Source: CAD feature listing. Evaluate the final solid. Frame: model axes, mm. A direction names the side the tool comes from. Give positions to 0.01 mm unless a question says otherwise; leave off trailing zeros. Loops run counter-clockwise (first coordinate to the right, second up) from the corner with the lowest first, then second, coordinate; pieces in that order, holes last. Notation, with made-up numbers: (43, 41) -> (89, 41) arc R12 ccw to (89, 57) -> close; hole circle Ø3 at (57.5, 22). An arc over 180 degrees is marked (long way). Return JSON: item names as keys, results as strings. Group by question number.
```python
from build123d import *

# Parameters (mm, degrees)
F4_T     = -1.2
F5_SIZE  = 0.5
F6_W     = 3.6
F6_H     = 11.6
F7_DEPTH = 5


with BuildPart() as f3:
    # F2 (on offset) → F3 section 0
    with BuildSketch(Plane.XY.offset(165)):
        with BuildLine():
            Line((-64, -36), (64, -36))
            ThreePointArc((64, -36), (89.4558441227, -25.4558441227), (100, 0))
            ThreePointArc((100, 0), (89.4558441227, 25.4558441227), (64, 36))
            Line((64, 36), (-64, 36))
            ThreePointArc((-64, 36), (-89.4558441227, 25.4558441227), (-100, 0))
            ThreePointArc((-100, 0), (-89.4558441227, -25.4558441227), (-64, -36))
        make_face()
    # F0 (on Top) → F3 section 1
    with BuildSketch(Plane.XY):
        with BuildLine():
            Line((-64, -36), (64, -36))
            ThreePointArc((64, -36), (89.4558441227, -25.4558441227), (100, 0))
            ThreePointArc((100, 0), (89.4558441227, 25.4558441227), (64, 36))
            Line((64, 36), (-64, 36))
            ThreePointArc((-64, 36), (-89.4558441227, 25.4558441227), (-100, 0))
            ThreePointArc((-100, 0), (-89.4558441227, -25.4558441227), (-64, -36))
        make_face()
    loft()

    # F4
    f4_openings = [f3.faces().sort_by_distance(p)[0] for p in [
        (0, 0, 0),
    ]]
    offset(amount=F4_T, openings=f4_openings)

    # F5
    f5_edges = [f3.edges().sort_by_distance(p)[0] for p in [
        (-100, 0, 165),
        (0, 36, 165),
        (100, 0, 165),
        (0, -36, 165),
        (-98.8, 0, 163.8),
        (0, -34.8, 163.8),
        (98.8, 0, 163.8),
        (0, 34.8, 163.8),
    ]]
    chamfer(f5_edges, length=F5_SIZE)

    # F6 (on face) → F7 (join)
    with BuildSketch(Plane(origin=(0, 0, 163.8), x_dir=(1, 0, 0), z_dir=(0, 0, -1))):
        Rectangle(F6_W, F6_H)
    extrude(amount=F7_DEPTH)


solid = f3.part
```
1) Mould query, pull axis X, two halves, no side actions, for faces 3 (the face through (1, 36, 81)), 4 (the face through (-1, -34.8, 81)), 5 (the face through (1, 8, 163.8)). Classes: released by +X, released by -X, zero draft, split by the parting line, or undercut.
2) Contact query for flat-ended pins moving along their axis: P1, Ø2, axis at x = 71, y = -8, coming from the -Z side; P2, Ø1, axis at y = 26.5, z = 102, coming from the +X side; P3, Ø1, axis at y = -10.5, z = 122.5, coming from the +X side. Output: stop coordinate, or through.
3) Cut plane B-B on x = 10.5. Return loops of the section in (y, z).
4) Reachability of faces 1 (the face through (1, 0, 165)), 2 (the face through (1.8, 0, 161)) from +Z, -Z, +X, -X, +Y, -Y: full face, straight path, thin tool, end or side. Return the list, or none.
5) Material intervals for line 1 (Y direction, x = 65, z = 136); line 2 (X direction, y = 28.5, z = 127); line 3 (Z direction, x = -29, y = -12.5), sorted ascending.
6) Cut plane A-A on z = 18.5. Return loops of the section in (x, y), then the cut area to 3 significant figures.
Calculated:
{
 "1": {"face 3": "zero draft", "face 4": "undercut", "face 5": "undercut"},
 "2": {"P1": "z = 163.8", "P2": "x = 88.9", "P3": "x = 98.58"},
 "3": {"outline": "(-36, 0) -> (-34.8, 0) -> (-34.8, 163.3) -> (-34.3, 163.8) -> (34.3, 163.8) -> (34.8, 163.3) -> (34.8, 0) -> (36, 0) -> (36, 164.5) -> (35.5, 165) -> (-35.5, 165) -> (-36, 164.5) -> close"},
 "4": {"face 1": "+Z, +X, -X, +Y, -Y", "face 2": "-Z"},
 "5": {"line 1": "-35.99 to -34.79, 34.79 to 35.99", "line 2": "-85.99 to -83.97, 83.97 to 85.99", "line 3": "163.8 to 165"},
 "6": {"outline": "(-64, -36) -> (64, -36) arc R36 ccw to (64, 36) -> (-64, 36) arc R36 ccw to start; hole (-64, -34.8) -> (64, -34.8) arc R34.8 ccw to (64, 34.8) -> (-64, 34.8) arc R34.8 ccw to start", "area": "574 mm2"}
}
